Design review of the part shown in the three views and the two pictorial views. Dimensions are in mm from the part's minimum x, y and z. A direction names the side the tool comes from. Round coordinates to 2 decimals unless told otherwise and drop trailing zeros. Order: outer loops, then holes, each group sorted by start corner. A loop starts at its lowest first (then second) coordinate and runs counter-clockwise, first axis right, second up. Notation, with made-up numbers: M 54.25,89.25 L 81.25,89.25 A24 ccw 81.25,120.25 Z; hole C 30,44.5 d2. An arc over 180 degrees is marked long. Use a Markdown table: item, result. Add a question column.
(1) The part is to be moulded in two halves that separate along X. For the marked faces 3, 4 and 5, say which applies: released by +X, released by -X, zero draft, split by the parting line, or undercut.
(2) For pin 1 (4 mm diameter, centred on x = 22, y = 34, fed in from -Z), flat-tipped, find the tip position at first contact; note if it passes through.
(3) Take a section at C-C (x = 101.6). Write out the cut boundary in (y, z).
(4) Take a section at A-A (y = 16.5). Write out the cut boundary in (x, z).
(5) To check wall thickness, follow probe 1 along Z at (x, y) = (86, 16.5); probe 2 along Z at (x, y) = (101, 95). State the ranges of each line that lie inside material, in increasing order. Write a range as from..to.
(6) Take a section at B-B (z = 101.6). Write out the cut boundary in (x, y), then the cut area to 3 significant figures.
(7) Machinability: for the marked faces 1 and 2, which of the approach directions +Z, -Z, +X, -X, +Y, -Y give a long, thin tool a straight path to every point of the face, cutting with its end or side? Answer none if there is none.
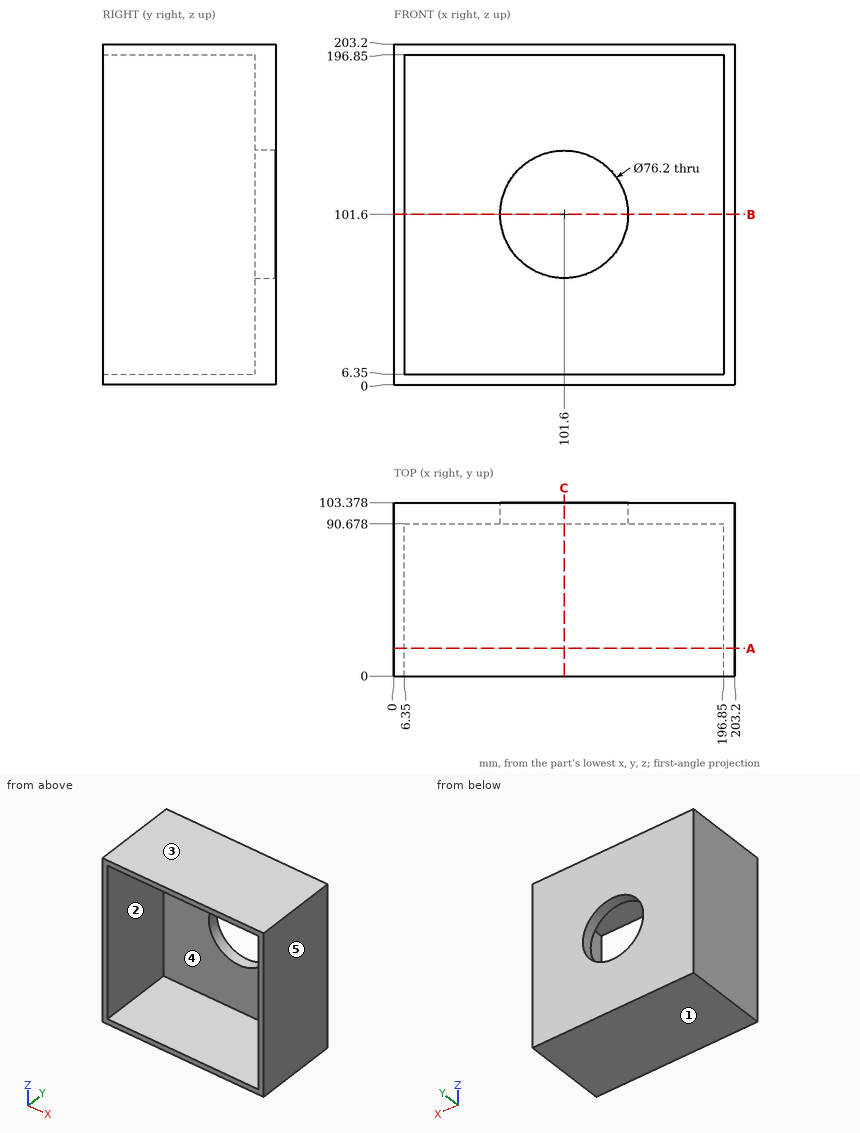
Verdict:
| question | item | result |
|---|---|---|
| 1 | face 3 | zero draft |
| 1 | face 4 | undercut |
| 1 | face 5 | released by +X |
| 2 | pin 1 | stops at z = 0 |
| 3 | outline | M 0,0 L 103.38,0 L 103.38,63.5 L 90.68,63.5 L 90.68,6.35 L 0,6.35 Z; M 0,196.85 L 90.68,196.85 L 90.68,139.7 L 103.38,139.7 L 103.38,203.2 L 0,203.2 Z |
| 4 | outline | M 0,0 L 203.2,0 L 203.2,203.2 L 0,203.2 Z; hole M 6.35,6.35 L 196.85,6.35 L 196.85,196.85 L 6.35,196.85 Z |
| 5 | probe 1 | z = 0..6.35, 196.85..203.2 |
| 5 | probe 2 | z = 0..63.5, 139.7..203.2 |
| 6 | outline | M 0,0 L 6.35,0 L 6.35,90.68 L 63.5,90.68 L 63.5,103.38 L 0,103.38 Z; M 139.7,90.68 L 196.85,90.68 L 196.85,0 L 203.2,0 L 203.2,103.38 L 139.7,103.38 Z |
| 6 | area | 2,760 mm^2 |
| 7 | face 1 | -Z, +X, -X, +Y, -Y |
| 7 | face 2 | -Y |
